Verification items for this drawing (mm, ordinates from the low corner). A direction names the side the tool comes from. Coordinates: 2 decimals unless noted, no trailing zeros. Order: outer loops, then holes, each group sorted by start corner. A loop starts at its lowest first (then second) coordinate and runs counter-clockwise, first axis right, second up. Notation, with made-up numbers: (27.5, 24.25) -> (48.5, 24.25) arc R17 ccw to (48.5, 52.25) -> close; hole circle Ø7 at (4.5, 25). An arc over 180 degrees is marked (long way). Answer as CSV lines item,"result". Start each with the question number.
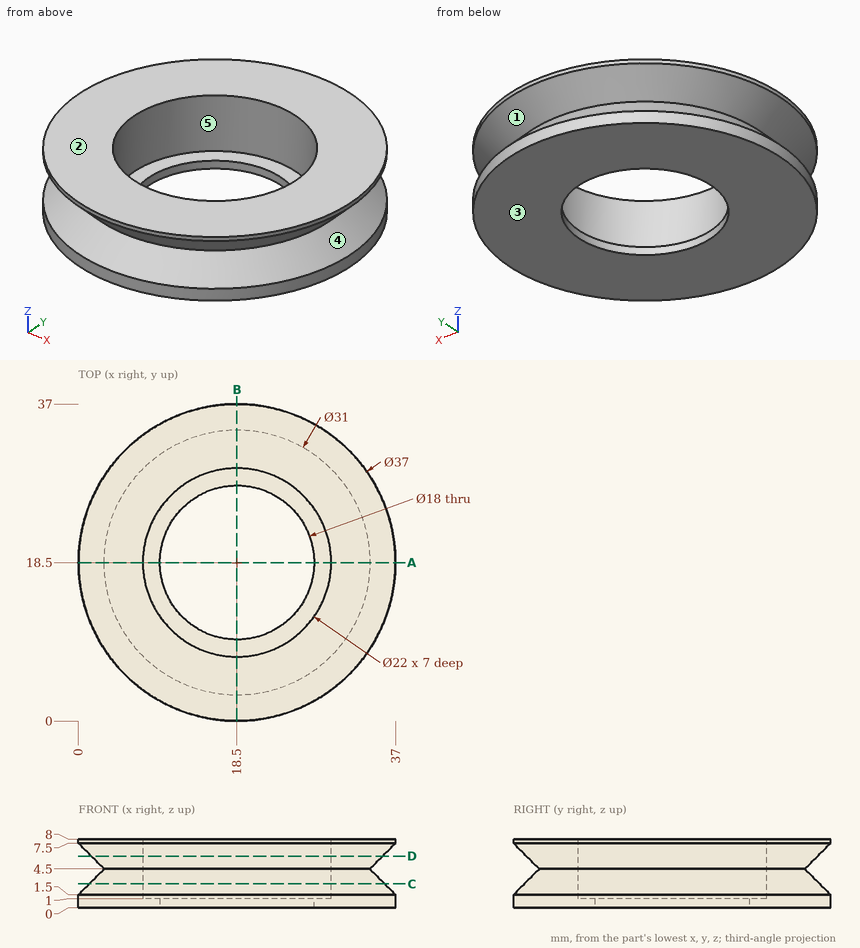
Q1. Go/stop test with flat-tipped pins: pin 1 Ø1.5 at (x, y) = (26.5, 19) entering from -Z; pin 2 Ø1.5 at (y, z) = (28, 2) entering from -X; pin 3 Ø20.5 at (x, y) = (18.5, 18.5) entering from +Z. Record where each tip stops, or that it passes through.
Q2. Sectioned sample at C-C, the plane z = 2.75. Record the cut outline in (x, y).
Q3. Release check for a two-part mould opening along Z. For the marked faces 3, 4 and 5 record: released by +Z, released by -Z, zero draft, split by the parting line, or undercut.
Q4. Sectioned sample at A-A, the plane y = 18.5. Record the cut outline in (x, z).
Q5. Thickness scan on L1, parallel to X at y = 18.5, z = 0.6; L2, parallel to X at y = 18, z = 6.5. Record the ranges inside material, lowest first.
Q6. Sectioned sample at D-D, the plane z = 6. Record the cut outline in (x, y), then the cut area to 3 significant figures.
Q7. Access from +Z, -Z, +X, -X, +Y, -Y to the whole of each face (thin tool, end or side, straight path). Record for the marked faces 1 and 2.
Geometry results:
1,pin 1,"passes through"
1,pin 2,"stops at x = 2.3"
1,pin 3,"stops at z = 1"
2,outline,"circle Ø34.5 at (18.5, 18.5); hole circle Ø22 at (18.5, 18.5)"
3,face 3,"released by -Z"
3,face 4,"undercut"
3,face 5,"zero draft"
4,outline,"(0, 0) -> (9.5, 0) -> (9.5, 1) -> (7.5, 1) -> (7.5, 8) -> (0, 8) -> (0, 7.5) -> (3, 4.5) -> (0, 1.5) -> close; (27.5, 0) -> (37, 0) -> (37, 1.5) -> (34, 4.5) -> (37, 7.5) -> (37, 8) -> (29.5, 8) -> (29.5, 1) -> (27.5, 1) -> close"
5,L1,"x = 0 to 9.5, 27.5 to 37"
5,L2,"x = 1.01 to 7.51, 29.49 to 35.99"
6,outline,"circle Ø34 at (18.5, 18.5); hole circle Ø22 at (18.5, 18.5)"
6,area,"528 mm^2"
7,face 1,"none"
7,face 2,"+Z, +X, -X, +Y, -Y"
